from build123d import *

# Parameters (mm, degrees)
F1_DEPTH = 577.85
F2_R     = 5.08
F4_DEPTH = 76.2


with BuildPart() as f1:
    # F0 (on Front) → F1 (new body)
    with BuildSketch(Plane.XZ):
        Polygon((-38.1, -38.1), (-31.75, -38.1), (-31.75, 31.75), (38.1, 31.75), (38.1, 38.1), (-38.1, 38.1), align=None)
    extrude(amount=F1_DEPTH)

    # F2
    f2_edges = [f1.edges().sort_by_distance(p)[0] for p in [
        (-31.75, -288.925, 31.75),
        (38.1, -288.925, 31.75),
        (-31.75, -288.925, -38.1),
    ]]
    fillet(f2_edges, radius=F2_R)

    # F3 (on face) → F4 (cut)
    with BuildSketch(Plane.XY.offset(38.1)):
        Polygon((-38.1, -577.85), (38.1, -577.85), (-38.1, -547.063202), align=None)
    extrude(amount=-F4_DEPTH, mode=Mode.SUBTRACT)


solid = f1.part
For this review, take the finished solid that the model builds, in its own axes (mm). A direction names the side the tool comes from. Round coordinates to 2 decimals unless told otherwise and drop trailing zeros. Order: outer loops, then holes, each group sorted by start corner. A loop starts at its lowest first (then second) coordinate and runs counter-clockwise, first axis right, second up. Notation, with made-up numbers: (-36.75, 33.25) -> (0.25, 33.25) arc R22 cw to (0.25, 68.25) -> close; hole circle Ø6 at (52.25, 0). An arc over 180 degrees is marked (long way). Write item = value, one per line. Start each with the question number.
1) Take a section at A-A on y = -178. State the section outline as (x, z) points, plus the area to 3 significant figures.
2) Insertion check: pin 1 (6 mm diameter, centred on y = -302.5, z = -11, fed in from +X); pin 2 (18 mm diameter, centred on x = 2, y = -407, fed in from -Z). Each pin has a flat end and moves straight along its axis. Give the tip position at first contact, or say it passes through.
3) Tool access review of faces 1 (the face through (1, -285, 38.1)), 2 (the face through (3, -284, 31.75)): name each direction out of +Z, -Z, +X, -X, +Y, -Y from which nothing blocks a thin tool from reaching the whole face with its end or side.
4) To check wall thickness, follow line 1 (Z direction, x = -0.5, y = -176); line 2 (X direction, y = -266.5, z = -10); line 3 (X direction, y = -245, z = 27.5). State the ranges of each line that lie inside material, in increasing order. Write a range as from..to.
5) Take a section at C-C on x = -4. State the section outline as (y, z) points, plus the area to 3 significant figures.
6) Take a section at B-B on z = -10. State the section outline as (x, y) points.
Verdict:
q1.outline = (-38.1, -38.1) -> (-36.83, -38.1) arc R5.08 ccw to (-31.75, -33.02) -> (-31.75, 26.67) arc R5.08 cw to (-26.67, 31.75) -> (33.02, 31.75) arc R5.08 ccw to (38.1, 36.83) -> (38.1, 38.1) -> (-38.1, 38.1) -> close
q1.area = 922 mm2
q2.pin_1 = -31.75
q2.pin_2 = 31.75
q3.face_1 = +Z, +X, -X, +Y, -Y
q3.face_2 = -Z, +X, +Y, -Y
q4.line_1 = 31.75..38.1
q4.line_2 = -38.1..-31.75
q4.line_3 = -38.1..-31.68
q5.outline = (-560.84, 31.75) -> (0, 31.75) -> (0, 38.1) -> (-560.84, 38.1) -> close
q5.area = 3,560 mm2
q6.outline = (-38.1, -547.06) -> (-31.75, -549.63) -> (-31.75, 0) -> (-38.1, 0) -> close
